```python
from build123d import *

# Parameters (mm, degrees)
SKETCH_1_W               = 70
SKETCH_1_H               = 95
EXTRUDE_1_DEPTH          = 20
SHELL_1_T                = -3
SKETCH_2_W               = 60
SKETCH_2_H               = 76
CUT_EXTRUDE_1_DEPTH      = 1
SKETCH_3_W               = 50
SKETCH_3_H               = 70
CUT_EXTRUDE_2_DEPTH      = 20
SKETCH_4_R               = 1.35
EXTRUDE_2_DEPTH          = 3
SKETCH_5_W               = 5
SKETCH_5_H               = 7
EXTRUDE_3_DEPTH          = 6
SKETCH_6_W               = 2.5
SKETCH_6_H               = 5.5
CUT_EXTRUDE_3_DEPTH      = 6.2
SKETCH_7_R               = 1.6
CUT_EXTRUDE_4_DEPTH      = 6.2
MIRROR_2_COPY_1_SKETCH_W = 5
MIRROR_2_COPY_1_SKETCH_H = 7
MIRROR_2_COPY_1_DEPTH    = 6
MIRROR_4_COPY_1_SKETCH_W = 2.5
MIRROR_4_COPY_1_SKETCH_H = 5.5
MIRROR_4_COPY_1_DEPTH    = 6.2
MIRROR_6_COPY_1_SKETCH_R = 1.6
MIRROR_6_COPY_1_DEPTH    = 6.2
EXTRUDE_4_DEPTH          = 70
SKETCH_9_R               = 1.6
CUT_EXTRUDE_5_DEPTH      = 70
SKETCH_10_W              = 60
SKETCH_10_H              = 12
CUT_EXTRUDE_6_DEPTH      = 30
SKETCH_11_W              = 3
SKETCH_11_H              = 7
CUT_EXTRUDE_7_DEPTH      = 2
SKETCH_12_R              = 3
CUT_EXTRUDE_8_DEPTH      = 0.5
CUT_EXTRUDE_9_DEPTH      = 0.5
SKETCH_14_W              = 20
SKETCH_14_H              = 10
CUT_EXTRUDE_10_DEPTH     = 10
FILLET_1_R               = 3
CHAMFER_1_SIZE           = 0.2


with BuildPart() as part:
    # 草图1 → 凸台-拉伸1 (new body)
    with BuildSketch(Plane.XY):
        Rectangle(SKETCH_1_W, SKETCH_1_H)
    extrude(amount=EXTRUDE_1_DEPTH)

    # 抽壳1
    shell_1_openings = [part.faces().sort_by_distance(p)[0] for p in [
        (0, 0, 0),
    ]]
    offset(amount=SHELL_1_T, openings=shell_1_openings, kind=Kind.INTERSECTION)

    # 草图2 → 切除-拉伸1 (cut)
    with BuildSketch(Plane.XY.offset(20)):
        Rectangle(SKETCH_2_W, SKETCH_2_H)
    extrude(amount=-CUT_EXTRUDE_1_DEPTH, mode=Mode.SUBTRACT)

    # 草图3 → 切除-拉伸2 (cut)
    with BuildSketch(Plane.XY.offset(19)):
        with Locations((0, 1)):
            Rectangle(SKETCH_3_W, SKETCH_3_H)
    extrude(amount=-CUT_EXTRUDE_2_DEPTH, mode=Mode.SUBTRACT)

    # 草图4 → 凸台-拉伸2 (add)
    # profile 1 of 4: a face of its own
    with BuildSketch(Plane.XY.offset(10)):
        with BuildLine():
            Line((20.5, 33), (32, 33))
            Line((32, 33), (32, 28))
            Line((32, 28), (20.5, 28))
            ThreePointArc((20.5, 28), (18, 30.5), (20.5, 33))
        make_face()
        with Locations((20.5, 30.5)):
            Circle(SKETCH_4_R, mode=Mode.SUBTRACT)
    # profile 2 of 4: a face of its own
    with BuildSketch(Plane.XY.offset(10)):
        with BuildLine():
            Line((-20.5, 33), (-32, 33))
            Line((-32, 33), (-32, 28))
            Line((-32, 28), (-20.5, 28))
            ThreePointArc((-20.5, 28), (-18, 30.5), (-20.5, 33))
        make_face()
        with Locations((-20.5, 30.5)):
            Circle(SKETCH_4_R, mode=Mode.SUBTRACT)
    # profile 3 of 4: a face of its own
    with BuildSketch(Plane.XY.offset(10)):
        with BuildLine():
            Line((-20.5, -27), (-32, -27))
            Line((-32, -27), (-32, -32))
            Line((-32, -32), (-20.5, -32))
            ThreePointArc((-20.5, -32), (-18, -29.5), (-20.5, -27))
        make_face()
        with Locations((-20.5, -29.5)):
            Circle(SKETCH_4_R, mode=Mode.SUBTRACT)
    # profile 4 of 4: a face of its own
    with BuildSketch(Plane.XY.offset(10)):
        with BuildLine():
            Line((20.5, -27), (32, -27))
            Line((32, -27), (32, -32))
            Line((32, -32), (20.5, -32))
            ThreePointArc((20.5, -32), (18, -29.5), (20.5, -27))
        make_face()
        with Locations((20.5, -29.5)):
            Circle(SKETCH_4_R, mode=Mode.SUBTRACT)
    extrude(amount=-EXTRUDE_2_DEPTH)

    # 草图5 → 凸台-拉伸3 (add)
    with BuildSketch(Plane(origin=(-32, 0, 0), x_dir=(0, 0, -1), z_dir=(1, 0, 0))):
        with Locations((-2.5, 41)):
            Rectangle(SKETCH_5_W, SKETCH_5_H)
    extrude_3 = extrude(amount=EXTRUDE_3_DEPTH)

    # 草图6 → 切除-拉伸3 (cut)
    with BuildSketch(Plane(origin=(-26, 0, 0), x_dir=(0, 0, -1), z_dir=(1, 0, 0))):
        with Locations((-3.05, 41.5)):
            Rectangle(SKETCH_6_W, SKETCH_6_H)
    cut_extrude_3 = extrude(amount=-CUT_EXTRUDE_3_DEPTH, mode=Mode.SUBTRACT)

    # 草图7 → 切除-拉伸4 (cut)
    with BuildSketch(Plane(origin=(0, 0, 0), x_dir=(-1, 0, 0), z_dir=(0, 0, -1))):
        with Locations((29, 41.5)):
            Circle(SKETCH_7_R)
    cut_extrude_4 = extrude(amount=-CUT_EXTRUDE_4_DEPTH, mode=Mode.SUBTRACT)

    # 镜向1: 凸台-拉伸3 across plane
    add(extrude_3.mirror(Plane.ZX))

    # 镜向2: 凸台-拉伸3 across plane
    add(extrude_3.mirror(Plane(origin=(0, 0, 0), x_dir=(0, 0, 1), z_dir=(1, 0, 0))))

    # 镜向2 copy 1 sketch → 镜向2 copy 1 (add)
    with BuildSketch(Plane(origin=(32, 0, 0), x_dir=(0, 0, -1), z_dir=(-1, 0, 0))):
        with Locations((-2.5, 41)):
            Rectangle(MIRROR_2_COPY_1_SKETCH_W, MIRROR_2_COPY_1_SKETCH_H)
    extrude(amount=MIRROR_2_COPY_1_DEPTH)

    # 镜向3: 切除-拉伸3 across plane
    add(cut_extrude_3.mirror(Plane.ZX), mode=Mode.SUBTRACT)

    # 镜向4: 切除-拉伸3 across plane
    add(cut_extrude_3.mirror(Plane(origin=(0, 0, 0), x_dir=(0, 0, 1), z_dir=(1, 0, 0))), mode=Mode.SUBTRACT)

    # 镜向4 copy 1 sketch → 镜向4 copy 1 (cut)
    with BuildSketch(Plane(origin=(26, 0, 0), x_dir=(0, 0, -1), z_dir=(-1, 0, 0))):
        with Locations((-3.05, 41.5)):
            Rectangle(MIRROR_4_COPY_1_SKETCH_W, MIRROR_4_COPY_1_SKETCH_H)
    extrude(amount=-MIRROR_4_COPY_1_DEPTH, mode=Mode.SUBTRACT)

    # 镜向5: 切除-拉伸4 across plane
    add(cut_extrude_4.mirror(Plane.ZX), mode=Mode.SUBTRACT)

    # 镜向6: 切除-拉伸4 across plane
    add(cut_extrude_4.mirror(Plane(origin=(0, 0, 0), x_dir=(0, 0, 1), z_dir=(1, 0, 0))), mode=Mode.SUBTRACT)

    # 镜向6 copy 1 sketch → 镜向6 copy 1 (cut)
    with BuildSketch(Plane(origin=(0, 0, 0), x_dir=(1, 0, 0), z_dir=(0, 0, -1))):
        with Locations((29, 41.5)):
            Circle(MIRROR_6_COPY_1_SKETCH_R)
    extrude(amount=-MIRROR_6_COPY_1_DEPTH, mode=Mode.SUBTRACT)

    # 草图8 → 凸台-拉伸4 (add)
    with BuildSketch(Plane(origin=(35, 0, 0), x_dir=(0, 0, -1), z_dir=(1, 0, 0))):
        with BuildLine():
            Line((-15.706419427, 57.062257962), (-10, 47.5))
            Line((-10, 47.5), (-20, 47.5))
            Line((-20, 47.5), (-20, 49.5))
            ThreePointArc((-20, 49.5), (-24.348062201, 56.968674765), (-15.706419427, 57.062257962))
        make_face()
    extrude(amount=-EXTRUDE_4_DEPTH)

    # 草图9 → 切除-拉伸5 (cut)
    with BuildSketch(Plane(origin=(35, 0, 0), x_dir=(0, 0, -1), z_dir=(1, 0, 0))):
        with Locations((-20, 54.5)):
            Circle(SKETCH_9_R)
    extrude(amount=-CUT_EXTRUDE_5_DEPTH, mode=Mode.SUBTRACT)

    # 草图10 → 切除-拉伸6 (cut)
    with BuildSketch(Plane(origin=(0, 0, 0), x_dir=(-1, 0, 0), z_dir=(0, 0, -1))):
        with Locations((0, 53.5)):
            Rectangle(SKETCH_10_W, SKETCH_10_H)
    extrude(amount=-CUT_EXTRUDE_6_DEPTH, mode=Mode.SUBTRACT)

    # 草图11 → 切除-拉伸7 (cut)
    with BuildSketch(Plane(origin=(-30, 0, 0), x_dir=(0, 0, -1), z_dir=(1, 0, 0))):
        with Locations((-20, 61)):
            Rectangle(SKETCH_11_W, SKETCH_11_H)
    cut_extrude_7 = extrude(amount=-CUT_EXTRUDE_7_DEPTH, mode=Mode.SUBTRACT)

    # 镜向7: 切除-拉伸7 across plane
    add(cut_extrude_7.mirror(Plane(origin=(0, 0, 0), x_dir=(0, 0, 1), z_dir=(1, 0, 0))), mode=Mode.SUBTRACT)

    # 草图12 → 切除-拉伸8 (cut)
    with BuildSketch(Plane(origin=(35, 0, 0), x_dir=(0, 0, -1), z_dir=(1, 0, 0))):
        with Locations((-20, 54.5)):
            Circle(SKETCH_12_R)
    cut_extrude_8 = extrude(amount=-CUT_EXTRUDE_8_DEPTH, mode=Mode.SUBTRACT)

    # 镜向8: 切除-拉伸8 across plane
    add(cut_extrude_8.mirror(Plane(origin=(0, 0, 0), x_dir=(0, 0, 1), z_dir=(1, 0, 0))), mode=Mode.SUBTRACT)

    # 草图13 → 切除-拉伸9 (cut)
    with BuildSketch(Plane.XY.offset(20)):
        Polygon((35, 49.5), (30, 49.5), (30, 47.5), (-30, 47.5), (-30, 49.5), (-35, 49.5), (-35, -47.5), (35, -47.5), align=None)
    extrude(amount=-CUT_EXTRUDE_9_DEPTH, mode=Mode.SUBTRACT)

    # 草图14 → 切除-拉伸10 (cut)
    with BuildSketch(Plane(origin=(0, 47.5, 0), x_dir=(1, 0, 0), z_dir=(0, 1, 0))):
        with Locations((0, -11.5)):
            Rectangle(SKETCH_14_W, SKETCH_14_H)
    extrude(amount=-CUT_EXTRUDE_10_DEPTH, mode=Mode.SUBTRACT)

    # 圆角1
    fillet_1_edges = [part.edges().sort_by_distance(p)[0] for p in [
        (-35, 47.5, 5),
        (35, 47.5, 5),
        (35, -47.5, 9.75),
        (-35, -47.5, 9.75),
    ]]
    fillet(fillet_1_edges, radius=FILLET_1_R)

    # 倒角1
    chamfer_1_edges = [part.edges().sort_by_distance(p)[0] for p in [
        (0, 38, 19.5),
        (-30, 0, 19.5),
        (0, -38, 19.5),
        (30, 0, 19.5),
        (-35, 50.781128981, 11.95806244),
        (35, 50.781128981, 11.95806244),
        (-30, 53.741211504, 24.942088629),
        (-35, 56.968674765, 24.348062201),
        (30, 53.741211504, 24.942088629),
        (35, 56.968674765, 24.348062201),
        (-30, 49.5, 19.75),
        (-35, 49.5, 19.75),
        (30, 49.5, 19.75),
        (35, 49.5, 19.75),
        (-32.5, 49.5, 19.5),
        (-30, 48.5, 19.5),
        (0, 47.5, 19.5),
        (30, 48.5, 19.5),
        (32.5, 49.5, 19.5),
        (35, 2.5, 19.5),
        (34.121320344, -46.621320344, 19.5),
        (0, -47.5, 19.5),
        (-34.121320344, -46.621320344, 19.5),
        (-35, 2.5, 19.5),
    ]]
    chamfer(chamfer_1_edges, length=CHAMFER_1_SIZE)


solid = part.part
```
The model under review builds one solid part; all positions refer to its coordinate system, in mm. A direction names the side the tool comes from. Give positions to 0.01 mm unless a question says otherwise; leave off trailing zeros. Write each loop counter-clockwise with the first axis right and the second up, starting at its lowest first coordinate (ties: lowest second). Pieces come first, ordered by that corner, then holes. Notation, with made-up numbers: (-1, -16) - (38, -16) arc R26 cw to (38, 5) - close; hole circle Ø4 at (21, 47). An arc over 180 degrees is marked (long way). Answer in a Markdown table with one row per item. Add a question column.
1. We need section B-B on x = -23.5. Write out the cut boundary in (y, z).
2. We need section D-D on y = 54.5. State how many separate pieces and enclosed holes the cut face has, then the cut area to 3 significant figures.
3. We need section C-C on x = -7. Write out the cut boundary in (y, z), then the cut area to 3 significant figures.
4. Insertion check: P1, Ø4.5, axis at x = -20.5, y = -29.5, coming from the -Z side; P2, Ø1.5, axis at x = 25.5, y = 30, coming from the +Z side; P3, Ø2.5, axis at x = -23, y = -29.5, coming from the +Z side. Each pin has a flat end and moves straight along its axis. Give the tip position at first contact, or say it passes through.
5. Wall thickness on line 1 along Y through (x, z) = (29, 0.55); line 2 along Y through (x, z) = (20.5, 8.8); line 3 along X through (y, z) = (-23.5, 14.75): over which ranges is each line inside the solid? List them lowest first. Write a range as [from, to].
6. We need section A-A on y = 19. Write out the cut boundary in (x, z), then the cut area to 3 significant figures.
7. Tool access review of faces 1 (the flat face through (26, -27, 9)), 2 (the flat face through (30, 53, 17)), 3 (the flat face through (-29.1, 39.6, 1.8)): name each direction out of +Z, -Z, +X, -X, +Y, -Y from which nothing blocks a thin tool from reaching the whole face with its end or side.
8. Draft analysis for pull direction Y (two halves, no side actions). For faces 4 (the cylindrical face through (-32.37, 56.84, 24.42)), 5 (the flat face through (-31, 57.5, 20)), 6 (the flat face through (-29.1, -39.6, 1.8)), state which applies: +Y half, -Y half, draft (parallel to the pull), parting line (faces both ways), or undercut.
Ans:
| question | item | result |
|---|---|---|
| 1 | outline | (-47.5, 0) - (-44.5, 0) - (-44.5, 17) - (-34, 17) - (-34, 19) - (-38, 19) - (-38, 19.3) - (-38.2, 19.5) - (-47.3, 19.5) - (-47.5, 19.3) - close; (-32, 7) - (-27, 7) - (-27, 10) - (-32, 10) - close; (28, 7) - (33, 7) - (33, 10) - (28, 10) - close; (36, 17) - (44.5, 17) - (44.5, 0) - (47.5, 0) - (47.5, 19.3) - (47.3, 19.5) - (38.2, 19.5) - (38, 19.3) - (38, 19) - (36, 19) - close |
| 2 | separate pieces | 4 |
| 2 | enclosed holes | 0 |
| 2 | area | 73.3 mm^2 |
| 3 | outline | (-47.5, 0) - (-44.5, 0) - (-44.5, 17) - (-34, 17) - (-34, 19) - (-38, 19) - (-38, 19.3) - (-38.2, 19.5) - (-47.3, 19.5) - (-47.5, 19.3) - close; (36, 17) - (44.5, 17) - (44.5, 16.5) - (47.5, 16.5) - (47.5, 19.3) - (47.3, 19.5) - (38.2, 19.5) - (38, 19.3) - (38, 19) - (36, 19) - close; (44.5, 0) - (47.5, 0) - (47.5, 6.5) - (44.5, 6.5) - close |
| 3 | area | 131 mm^2 |
| 4 | P1 | stops at z = 7 |
| 4 | P2 | stops at z = 19 |
| 4 | P3 | stops at z = 10 |
| 5 | line 1 | y = [-47.5, -43.1], [-39.9, -37.5], [37.5, 39.9], [43.1, 47.5] |
| 5 | line 2 | y = [-47.5, -44.5], [-32, -30.85], [-28.15, -27], [28, 29.15], [31.85, 33], [44.5, 47.5] |
| 5 | line 3 | x = [-35, -32], [32, 35] |
| 6 | outline | (-35, 0) - (-32, 0) - (-32, 17) - (-25, 17) - (-25, 19) - (-30, 19) - (-30, 19.3) - (-30.2, 19.5) - (-34.8, 19.5) - (-35, 19.3) - close; (25, 17) - (32, 17) - (32, 0) - (35, 0) - (35, 19.3) - (34.8, 19.5) - (30.2, 19.5) - (30, 19.3) - (30, 19) - (25, 19) - close |
| 6 | area | 147 mm^2 |
| 7 | face 1 | -Z |
| 7 | face 2 | +Z, -Z, +Y |
| 7 | face 3 | none |
| 8 | face 4 | parting line |
| 8 | face 5 | +Y half |
| 8 | face 6 | undercut |
